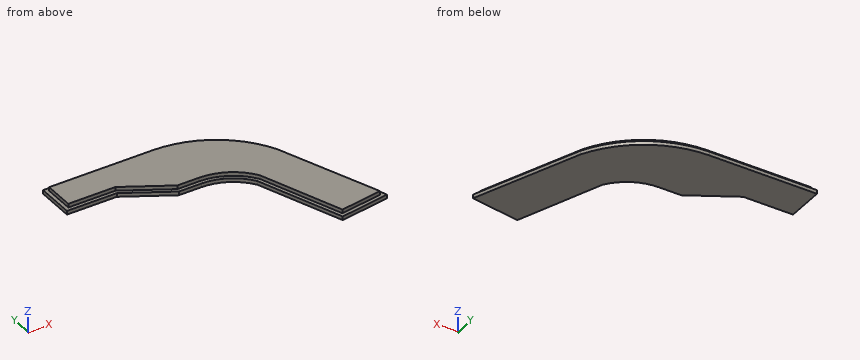
```python
from build123d import *

# Parameters (mm, degrees)
F1_DEPTH = 3
F3_DEPTH = 3


with BuildPart() as f1:
    # F0 (on Top) → F1 (new body)
    with BuildSketch(Plane.XY):
        with BuildLine():
            Line((-26.049673, 52.928504), (-112.191005, 52.928504))
            Line((-112.191005, 52.928504), (-112.191005, 22.928504))
            Line((-112.191005, 22.928504), (-72.191005, 22.928504))
            Line((-72.191005, 22.928504), (-35.867805, 1.957295))
            Line((-35.867805, 1.957295), (-17.654659, 1.957295))
            ThreePointArc((-17.654659, 1.957295), (1.351351, -2.846519), (15.792295, -16.104127))
            Line((15.792295, -16.104127), (41.093565, -83.207551))
            Line((41.093565, -83.207551), (80.600171, -76.944318))
            Line((80.600171, -76.944318), (48.117351, 6.989384))
            ThreePointArc((48.117351, 6.989384), (17.57128, 40.513403), (-26.049673, 52.928504))
        make_face()
    extrude(amount=F1_DEPTH)

    # F2 (on face) → F3 (join)
    with BuildSketch(Plane.XY.offset(3)):
        with BuildLine():
            Line((-35.063957, 4.957295), (-17.654659, 4.957295))
            ThreePointArc((-17.654659, 4.957295), (2.924994, -0.287204), (18.484649, -14.741409))
            Line((18.484649, -14.741409), (43.038213, -79.861787))
            Line((43.038213, -79.861787), (76.46174, -74.562943))
            Line((76.46174, -74.562943), (45.370091, 5.776055))
            ThreePointArc((45.370091, 5.776055), (15.933126, 37.999173), (-26.049673, 49.928504))
            Line((-26.049673, 49.928504), (-109.191005, 49.928504))
            Line((-109.191005, 49.928504), (-109.191005, 25.928504))
            Line((-109.191005, 25.928504), (-71.387158, 25.928504))
            Line((-71.387158, 25.928504), (-35.063957, 4.957295))
        make_face()
    extrude(amount=F3_DEPTH)


solid = f1.part
```
CAD build for the part. Positions are in the model's coordinates, mm. Round coordinates to 2 decimals unless told otherwise and drop trailing zeros. Write each loop counter-clockwise with the first axis right and the second up, starting at its lowest first coordinate (ties: lowest second). Pieces come first, ordered by that corner, then holes. Notation, with made-up numbers: (18, 59) - (32, 59) arc R17 cw to (32, 78) - close; hole circle Ø8 at (62, -0.75). An arc over 180 degrees is marked (long way). Return JSON: item names as keys, results as strings. Group by question number.
Item 1: Flat gauge pins, fed straight in: pin 1 Ø1.5 at (y, z) = (-37.5, 2.5) entering from -X; pin 2 Ø2.5 at (x, z) = (-25.5, 1) entering from -Y; pin 3 Ø3.5 at (x, z) = (-65.5, 5) entering from +Y. Where does each tip first touch, or does it go through?
Item 2: Band-saw the part on C-C on y = -47.5. List the corners of the cut face in (x, z), plus the area to 3 significant figures.
Item 3: Band-saw the part on A-A on z = 1.9. List the corners of the cut face in (x, y), plus the area to 3 significant figures.
Item 4: Probe probe 1 along Y at (x, z) = (-32.5, 4.8); probe 2 along Y at (x, z) = (-98.5, 2.6); probe 3 along X at (y, z) = (-28, 2.8). List the from-to ranges inside material, lowest first.
Item 5: Band-saw the part on B-B on x = -98. List the corners of the cut face in (y, z), plus the area to 3 significant figures.
Resolved:
{
 "1": {"pin 1": "stops at x = 23.58", "pin 2": "stops at y = 1.96", "pin 3": "stops at y = 49.93"},
 "2": {"outline": "(27.63, 0) - (69.21, 0) - (69.21, 3) - (65.99, 3) - (65.99, 6) - (30.84, 6) - (30.84, 3) - (27.63, 3) - close", "area": "230 mm²"},
 "3": {"outline": "(-112.19, 22.93) - (-72.19, 22.93) - (-35.87, 1.96) - (-17.65, 1.96) arc R40 cw to (15.79, -16.1) - (41.09, -83.21) - (80.6, -76.94) - (48.12, 6.99) arc R82.84 ccw to (-26.05, 52.93) - (-112.19, 52.93) - close", "area": "9,510 mm²"},
 "4": {"probe 1": "y = 4.96 to 49.93", "probe 2": "y = 22.93 to 52.93", "probe 3": "x = 20.28 to 61.66"},
 "5": {"outline": "(22.93, 0) - (52.93, 0) - (52.93, 3) - (49.93, 3) - (49.93, 6) - (25.93, 6) - (25.93, 3) - (22.93, 3) - close", "area": "162 mm²"}
}
